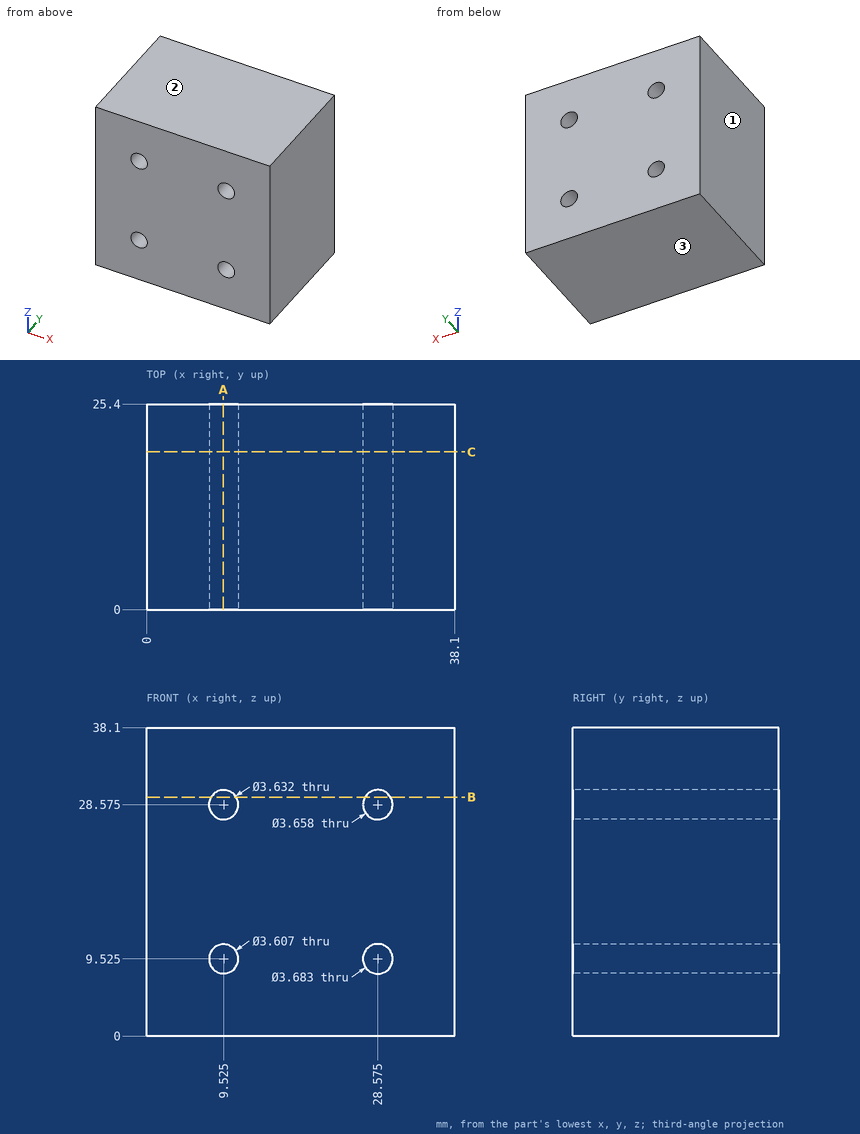
Input: dimensioned drawing with shaded views. Units: mm. Origin: part minimum x, y, z. Round coordinates to 2 decimals unless told otherwise and drop trailing zeros. Order: outer loops, then holes, each group sorted by start corner. A loop starts at its lowest first (then second) coordinate and runs counter-clockwise, first axis right, second up. Notation, with made-up numbers: (-28.75, -27) - (6.25, -27) arc R19 cw to (6.25, 9) - close; hole circle Ø6 at (68.25, 8). An arc over 180 degrees is marked (long way). Write item = value, one per line. Start each with the question number.
Q1. Cut plane C-C on y = 19.5. Return the cut outline in (x, z) (1 decimal), and give its area (3 significant figures).
Q2. Cut plane B-B on z = 29.5. Return the cut outline in (x, y).
Q3. Cut plane A-A on x = 9.5. Return the cut outline in (y, z).
Q4. Ray query, line 1 (X direction, y = 17.75, z = 27.5) (1 decimal); line 2 (Z direction, x = 30, y = 5.75). Return the intervals inside material, ascending. Write a range as from..to.
Q5. Pull-direction query (Z, two-part tool) for the marked faces 1, 2 and 3; classes: +Z half, -Z half, draft (parallel to the pull), parting line (faces both ways), or undercut.
Outcome:
q1.outline = (0, 0) - (38.1, 0) - (38.1, 38.1) - (0, 38.1) - close; hole circle Ø3.6 at (9.5, 9.5); hole circle Ø3.6 at (9.5, 28.6); hole circle Ø3.7 at (28.6, 9.5); hole circle Ø3.7 at (28.6, 28.6)
q1.area = 1,410 mm^2
q2.outline = (0, 0) - (7.96, 0) - (7.96, 25.4) - (0, 25.4) - close; (11.09, 0) - (27, 0) - (27, 25.4) - (11.09, 25.4) - close; (30.15, 0) - (38.1, 0) - (38.1, 25.4) - (30.15, 25.4) - close
q3.outline = (0, 0) - (25.4, 0) - (25.4, 7.72) - (0, 7.72) - close; (0, 11.33) - (25.4, 11.33) - (25.4, 26.76) - (0, 26.76) - close; (0, 30.39) - (25.4, 30.39) - (25.4, 38.1) - (0, 38.1) - close
q4.line_1 = 0..8.1, 11..27.1, 30.1..38.1
q4.line_2 = 0..8.36, 10.69..27.43, 29.72..38.1
q5.face_1 = draft
q5.face_2 = +Z half
q5.face_3 = -Z half
